Part model, mm, in its own coordinate system. Face numbers are marked on the shaded views. A direction names the side the tool comes from. Round coordinates to 2 decimals unless told otherwise and drop trailing zeros. Write each loop counter-clockwise with the first axis right and the second up, starting at its lowest first coordinate (ties: lowest second). Pieces come first, ordered by that corner, then holes.
1) Saw through at B-B on x = 8.5. Write the cut outline in (y, z).
2) Flat gauge pins, fed straight in: pin 1 (2 mm diameter, centred on x = -26.5, y = 6.5, fed in from +Z); pin 2 (5 mm diameter, centred on x = -33.94, z = -33.94, fed in from +Y); pin 3 (1 mm diameter, centred on x = 26, y = 6, fed in from -Z). Where does each tip first touch, or does it go through?
3) Pull direction Z, two halves, no side cores. Call the marked faces 1, 2 and 3: +Z half, -Z half, draft (parallel to the pull), parting line (faces both ways), or undercut.
4) Saw through at A-A on z = -4. Write the cut outline in (x, y), and give its area (3 significant figures).
5) Which spindle directions (+Z, -Z, +X, -X, +Y, -Y) get a long thin tool onto all of the face, cutting with end or side? Do the marked faces 4, 5, 6, 7 and 8. Say none if no direction does.
6) Saw through at C-C on y = 4.75. Count the separate pieces of the cut face and the enclosed holes in it, and give its area (3 significant figures).
7) Drill centre lines: L1, parallel to X at y = 3.5, z = 0; L2, parallel to X at y = 3.75, z = -8.5; L3, parallel to X at y = 0.75, z = -35 (1 decimal). Where is each one in solid material? Low to high.
Autodesk Inventor part; units mm, degrees
ref_plane "YZ Plane" through (0, 0, 0) normal (1, 0, 0) x (0, 1, 0)
ref_plane "XZ Plane" through (0, 0, 0) normal (0, 1, 0) x (-1, 0, 0)
ref_plane "XY Plane" through (0, 0, 0) normal (0, 0, 1) x (1, 0, 0)
sketch "Esquisse1" plane through (0, 0, 0) normal (0, 1, 0) x (-1, 0, 0)
  circle A0 centre (33.9411, 33.9411) radius 3
  line L0 (0, -58.8171) -> (0, 58.8171)
  line L1 (-58.8171, 0) -> (58.8171, 0)
  line L2 (0, 0) -> (33.9411, 33.9411) construction
  line L3 (26.6119, 35.0971) -> (33.234, 41.7193)
  line L4 (34.6482, 41.7193) -> (41.7193, 34.6482)
  line L5 (41.7193, 33.234) -> (35.0971, 26.6119)
  arc A1 (34.6482, 41.7193) -> (33.234, 41.7193) centre (33.9411, 41.0122) ccw
  arc A2 (41.7193, 33.234) -> (41.7193, 34.6482) centre (41.0122, 33.9411) ccw
  arc A3 (11.636, 24.364) -> (-11.636, 24.364) centre (0, 0) ccw construction
  arc A4 (13.7909, 28.8758) -> (-13.7909, 28.8758) centre (0, 0) ccw
  arc A5 (9.4812, 19.8521) -> (-9.4812, 19.8521) centre (0, 0) ccw
  arc A6 (9.4812, 19.8521) -> (13.7909, 28.8758) centre (11.636, 24.364) ccw
  arc A7 (-13.7909, 28.8758) -> (-9.4812, 19.8521) centre (-11.636, 24.364) ccw
  circle A8 centre (0, 0) radius 16
  arc A9 (20.5123, 34.3402) -> (0, 40) centre (0, 0) ccw
  arc A10 (40, 0) -> (34.3402, 20.5123) centre (0, 0) ccw
  arc A11 (20.5123, 34.3402) -> (26.6119, 35.0971) centre (23.0763, 38.6327) ccw
  arc A12 (35.0971, 26.6119) -> (34.3402, 20.5123) centre (38.6327, 23.0763) ccw
  circle A13 centre (-33.9411, 33.9411) radius 3
  line L6 (0, 0) -> (-33.9411, 33.9411) construction
  line L7 (-35.0971, 26.6119) -> (-41.7193, 33.234)
  line L8 (-41.7193, 34.6482) -> (-34.6482, 41.7193)
  line L9 (-33.234, 41.7193) -> (-26.6119, 35.0971)
  arc A14 (-41.7193, 34.6482) -> (-41.7193, 33.234) centre (-41.0122, 33.9411) ccw
  arc A15 (-33.234, 41.7193) -> (-34.6482, 41.7193) centre (-33.9411, 41.0122) ccw
  arc A16 (-24.364, 11.636) -> (-24.364, -11.636) centre (0, 0) ccw construction
  arc A17 (-28.8758, 13.7909) -> (-28.8758, -13.7909) centre (0, 0) ccw
  arc A18 (-19.8521, 9.4812) -> (-19.8521, -9.4812) centre (0, 0) ccw
  arc A19 (-19.8521, 9.4812) -> (-28.8758, 13.7909) centre (-24.364, 11.636) ccw
  arc A20 (-28.8758, -13.7909) -> (-19.8521, -9.4812) centre (-24.364, -11.636) ccw
  arc A21 (-34.3402, 20.5123) -> (-40, 0) centre (0, 0) ccw
  arc A22 (0, 40) -> (-20.5123, 34.3402) centre (0, 0) ccw
  arc A23 (-34.3402, 20.5123) -> (-35.0971, 26.6119) centre (-38.6327, 23.0763) ccw
  arc A24 (-26.6119, 35.0971) -> (-20.5123, 34.3402) centre (-23.0763, 38.6327) ccw
  circle A25 centre (-33.9411, -33.9411) radius 3
  line L10 (0, 0) -> (-33.9411, -33.9411) construction
  line L11 (-26.6119, -35.0971) -> (-33.234, -41.7193)
  line L12 (-34.6482, -41.7193) -> (-41.7193, -34.6482)
  line L13 (-41.7193, -33.234) -> (-35.0971, -26.6119)
  arc A26 (-34.6482, -41.7193) -> (-33.234, -41.7193) centre (-33.9411, -41.0122) ccw
  arc A27 (-41.7193, -33.234) -> (-41.7193, -34.6482) centre (-41.0122, -33.9411) ccw
  arc A28 (-11.636, -24.364) -> (11.636, -24.364) centre (0, 0) ccw construction
  arc A29 (-13.7909, -28.8758) -> (13.7909, -28.8758) centre (0, 0) ccw
  arc A30 (-9.4812, -19.8521) -> (9.4812, -19.8521) centre (0, 0) ccw
  arc A31 (-9.4812, -19.8521) -> (-13.7909, -28.8758) centre (-11.636, -24.364) ccw
  arc A32 (13.7909, -28.8758) -> (9.4812, -19.8521) centre (11.636, -24.364) ccw
  arc A33 (-20.5123, -34.3402) -> (0, -40) centre (0, 0) ccw
  arc A34 (-40, 0) -> (-34.3402, -20.5123) centre (0, 0) ccw
  arc A35 (-20.5123, -34.3402) -> (-26.6119, -35.0971) centre (-23.0763, -38.6327) ccw
  arc A36 (-35.0971, -26.6119) -> (-34.3402, -20.5123) centre (-38.6327, -23.0763) ccw
  circle A37 centre (33.9411, -33.9411) radius 3
  line L14 (0, 0) -> (33.9411, -33.9411) construction
  line L15 (35.0971, -26.6119) -> (41.7193, -33.234)
  line L16 (41.7193, -34.6482) -> (34.6482, -41.7193)
  line L17 (33.234, -41.7193) -> (26.6119, -35.0971)
  arc A38 (41.7193, -34.6482) -> (41.7193, -33.234) centre (41.0122, -33.9411) ccw
  arc A39 (33.234, -41.7193) -> (34.6482, -41.7193) centre (33.9411, -41.0122) ccw
  arc A40 (24.364, -11.636) -> (24.364, 11.636) centre (0, 0) ccw construction
  arc A41 (28.8758, -13.7909) -> (28.8758, 13.7909) centre (0, 0) ccw
  arc A42 (19.8521, -9.4812) -> (19.8521, 9.4812) centre (0, 0) ccw
  arc A43 (19.8521, -9.4812) -> (28.8758, -13.7909) centre (24.364, -11.636) ccw
  arc A44 (28.8758, 13.7909) -> (19.8521, 9.4812) centre (24.364, 11.636) ccw
  arc A45 (34.3402, -20.5123) -> (40, 0) centre (0, 0) ccw
  arc A46 (0, -40) -> (20.5123, -34.3402) centre (0, 0) ccw
  arc A47 (34.3402, -20.5123) -> (35.0971, -26.6119) centre (38.6327, -23.0763) ccw
  arc A48 (26.6119, -35.0971) -> (20.5123, -34.3402) centre (23.0763, -38.6327) ccw
  circle A49 centre (0, 0) radius 16 construction
  point P0 (23.7216, 32.2069)
  point P1 (32.2069, 23.7216)
  point P2 (-32.2069, 23.7216)
  point P3 (-23.7216, 32.2069)
  point P4 (-23.7216, -32.2069)
  point P5 (-32.2069, -23.7216)
  point P6 (32.2069, -23.7216)
  point P7 (23.7216, -32.2069)
  dimension "d1" = 6
  dimension "d2" = 48
  dimension "d3" = 6
  dimension "d4" = 6
  dimension "d5" = 45
  dimension "d6" = 1
  dimension "d9" = 10
  dimension "d10" = 9
  dimension "d11" = 40
  dimension "d12" = 5
  dimension "d13" = 27
extrude "Extrusion1" add sketch "Esquisse1" along normal blind 8 contours A33 A35 L11 A26 L12 A27 L13 A36 A34 L1 A17 A20 A18 A8 L0 A30 A31 A29 | L0 A29 A32 A30 A8 L1 A42 A43 A41 A45 A47 L15 A38 L16 A39 L17 A48 A46 | L1 A18 A19 A17 A21 A23 L7 A14 L8 A15 L9 A24 A22 L0 A4 A7 A5 A8 | A8 L0 A5 A6 A4 A9 A11 L3 A1 L4 A2 L5 A12 A10 L1 A41 A44 A42
equation "\"d4\" = d3"
properties part number "Colossus_7kW_Stator"
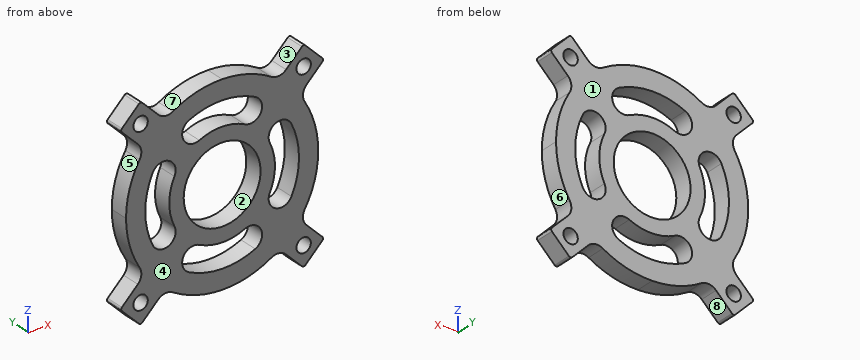
Completed:
1. outline: (0, -39.09) - (8, -39.09) - (8, -30.85) - (0, -30.85) - close; (0, -20.29) - (8, -20.29) - (8, -13.56) - (0, -13.56) - close; (0, 13.56) - (8, 13.56) - (8, 20.29) - (0, 20.29) - close; (0, 30.85) - (8, 30.85) - (8, 39.09) - (0, 39.09) - close
2. pin 1: stops at z = 35.99
2. pin 2: passes through
2. pin 3: stops at z = -34.99
3. face 1: draft
3. face 2: undercut
3. face 3: +Z half
4. outline: (-39.8, 0) - (-31.75, 0) - (-31.75, 8) - (-39.8, 8) - close; (-21.63, 0) - (-15.49, 0) - (-15.49, 8) - (-21.63, 8) - close; (15.49, 0) - (21.63, 0) - (21.63, 8) - (15.49, 8) - close; (31.75, 0) - (39.8, 0) - (39.8, 8) - (31.75, 8) - close
4. area: 227 mm2
5. face 4: +Z, -Z, +X, -X, -Y
5. face 5: -X, +Y, -Y
5. face 6: +X, +Y, -Y
5. face 7: +Z, +Y, -Y
5. face 8: -Z, +Y, -Y
6. separate pieces: 1
6. enclosed holes: 9
6. area: 3,540 mm2
7. L1: x = -40 to -32, -22 to -16, 16 to 22, 32 to 40
7. L2: x = -39.09 to -30.85, -20.29 to -13.56, 13.56 to 20.29, 30.85 to 39.09
7. L3: x = -41.4 to -36.7, -31.1 to -26.5, -19.4 to 19.4, 26.5 to 31.1, 36.7 to 41.4
